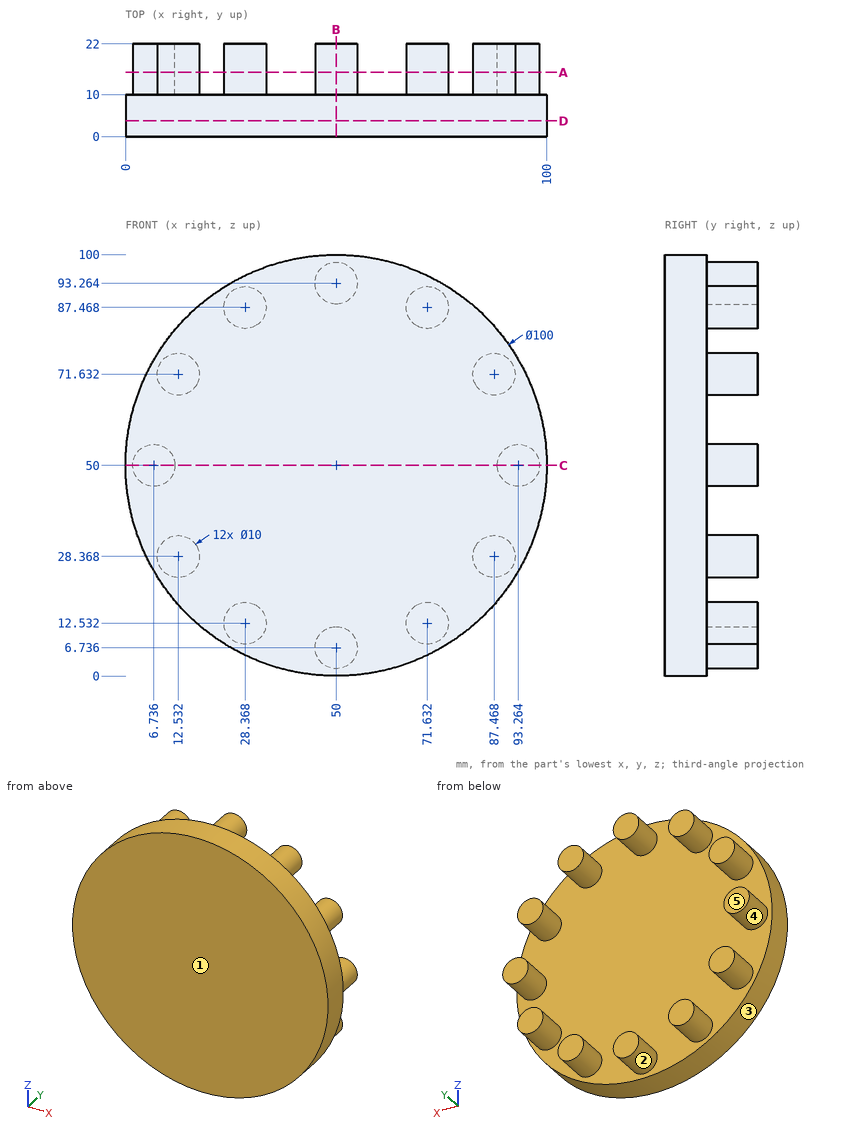
Answer from the drawing. Dimensions are ordinates in mm from the lowest x, y and z of the part. A direction names the side the tool comes from. Coordinates: 2 decimals unless noted, no trailing zeros. Write each loop counter-clockwise with the first axis right and the second up, starting at its lowest first coordinate (ties: lowest second). Pieces come first, ordered by that corner, then holes. Notation, with made-up numbers: M -25,62.5 L 0,62.5 A29 cw 0,90.5 Z; hole C 40.5,68.5 d3. An arc over 180 degrees is marked long. Write item = value, one per line.
1. Straight lines are drawn through the part: line 1 (Z direction, x = 89.5, y = 15.25); line 2 (Y direction, x = 68.5, z = 68.5); line 3 (Z direction, x = 14.5, y = 11.5). For each, find the intervals that lie inside material, in ascending order. Write a range as from..to.
Solution:
line_1 = 23.8..32.94, 46.71..53.29, 67.06..76.2
line_2 = 0..10
line_3 = 23.77..32.96, 67.04..76.23
2. The part is cut by section A-A (y = 15.25). State how many separate pieces and enclosed holes the cut face has.
Solution:
separate_pieces = 12
enclosed_holes = 0
3. Determine the mould class of the marked faces 3, 4 and 5 for opening direction Z: released by +Z, released by -Z, zero draft, split by the parting line, or undercut.
Solution:
face_3 = split by the parting line
face_4 = undercut
face_5 = zero draft
4. Flat-ended cylindrical pins translate along their axes: pin 1 (1.5 mm diameter, centred on y = 14, z = 74.5, fed in from +X); pin 2 (12 mm diameter, centred on y = 4, z = 53, fed in from -X); pin 3 (6 mm diameter, centred on x = 57.5, z = 80.5, fed in from +Y). Find the tip coordinate at first contact, or state that the pin passes through.
Solution:
pin_1 = 92
pin_2 = 0
pin_3 = 10
5. The part is cut by section D-D (y = 3.75). Determine the outline of the cut face in (x, z), then the cut area to 3 significant figures.
Solution:
outline = C 50,50 d100
area = 7,850 mm2
6. The part is cut by section B-B (x = 50). Determine the outline of the cut face in (y, z).
Solution:
outline = M 0,0 L 10,0 L 10,1.74 L 22,1.74 L 22,11.74 L 10,11.74 L 10,88.26 L 22,88.26 L 22,98.26 L 10,98.26 L 10,100 L 0,100 Z
7. For the marked faces 1 and 2, determine the directions among +Z, -Z, +X, -X, +Y, -Y from which every point of the face is accessible in a straight line to the end or side of a thin tool.
Solution:
face_1 = +Z, -Z, +X, -X, -Y
face_2 = +Y
8. The part is cut by section C-C (z = 50). Determine the outline of the cut face in (x, y), then the cut area to 3 significant figures.
Solution:
outline = M 0,0 L 100,0 L 100,10 L 98.26,10 L 98.26,22 L 88.26,22 L 88.26,10 L 11.74,10 L 11.74,22 L 1.74,22 L 1.74,10 L 0,10 Z
area = 1,240 mm2
